Verification items for the finished model (mm, model axes). A direction names the side the tool comes from. Give positions to 0.01 mm unless a question says otherwise; leave off trailing zeros. Order: outer loops, then holes, each group sorted by start corner. A loop starts at its lowest first (then second) coordinate and runs counter-clockwise, first axis right, second up. Notation, with made-up numbers: (-7.5, 8.5) -> (6.5, 8.5) arc R20 ccw to (6.5, 32.5) -> close; hole circle Ø10 at (5, -18.75). An arc over 180 degrees is marked (long way). Write each question's results on one line, items separated by ' | '. Start each with the question number.
1. Set-up check for faces 1 (the face through (5.01, -13.43, 0.81)), 2 (the face through (7, -12.522, 1)): record each of +Z, -Z, +X, -X, +Y, -Y from which the full face is reachable in a straight line by a thin tool's end or side.
2. Depth check by flat-ended pin: pin 1 Ø1.7 at (x, y) = (-15.04, -11.37) entering from -Z; pin 2 Ø0.5 at (y, z) = (4, 1) entering from +X; pin 3 Ø1.3 at (x, y) = (0, -13.97) entering from -Z; pin 4 Ø0.5 at (x, z) = (8, 1) entering from +Y. Enter the tip coordinate at first touch or a pass-through.
3. Cross-section at D-D, the plane x = -9. Enter the section's corners in (y, z).
4. Cross-section at A-A, the plane x = 10.16. Enter the section's corners in (y, z), then the cut area to 3 significant figures.
5. Material ranges on L1, parallel to Y at x = 2.54, z = 1.2; L2, parallel to Y at x = -22.5, z = 1.3; L3, parallel to Y at x = -20.95, z = 0.85, recorded low to high. Write a range as from..to.
6. Cross-section at B-B, the plane y = -13.97. State how many separate pieces and enclosed holes the cut face has, then the cut area to 3 significant figures.
7. Mould release check, pull along X, two halves, no side actions. Record for faces 3 (the face through (-13.64, -11.31, 0.79)), 4 (the face through (-18, 16.51, 1)), 5 (the face through (25.4, -20, 1)): +X half, -X half, draft (parallel to the pull), parting line (faces both ways), or undercut.
Autodesk Inventor part; units mm, degrees
ref_plane "YZ Plane" through (0, 0, 0) normal (1, 0, 0) x (0, 1, 0)
ref_plane "XZ Plane" through (0, 0, 0) normal (0, 1, 0) x (-1, 0, 0)
ref_plane "XY Plane" through (0, 0, 0) normal (0, 0, 1) x (1, 0, 0)
sketch "Sketch1" plane through (0, 0, 0) normal (0, 0, 1) x (1, 0, 0)
  line L0 (-25.4, -16.51) -> (25.4, -16.51)
  line L1 (25.4, -16.51) -> (25.4, 16.51)
  line L2 (25.4, 16.51) -> (-25.4, 16.51)
  line L3 (-25.4, 16.51) -> (-25.4, -10.64)
  line L4 (-10.0076, 16.51) -> (-10.0076, -12.5222)
  line L5 (-10.0076, -12.5222) -> (25.4, -12.5222)
  line L6 (-25.4, -16.51) -> (-25.4, -26.4922)
  line L7 (-25.4, -26.4922) -> (25.4, -26.4922)
  line L8 (25.4, -26.4922) -> (25.4, -16.51)
  circle A0 centre (-2.54, -13.97) radius 0.5461
  circle A1 centre (2.54, -13.97) radius 0.5461
  circle A2 centre (7.62, -13.97) radius 0.5461
  circle A3 centre (-5.08, -7.62) radius 0.4445
  circle A4 centre (0, -7.62) radius 0.4445
  circle A5 centre (5.08, -7.62) radius 0.4445
  circle A6 centre (10.16, -7.62) radius 0.4445
  circle A7 centre (-5.08, 10.16) radius 0.4445
  circle A8 centre (0, 10.16) radius 0.4445
  circle A9 centre (5.08, 10.16) radius 0.4445
  circle A10 centre (10.16, 10.16) radius 0.4445
  circle A11 centre (12.7, 10.16) radius 0.4445
  circle A12 centre (7.62, 10.16) radius 0.4445
  circle A13 centre (2.54, 10.16) radius 0.4445
  circle A14 centre (-2.54, 10.16) radius 0.4445
  circle A15 centre (12.7, -7.62) radius 0.4445
  circle A16 centre (7.62, -7.62) radius 0.4445
  circle A17 centre (2.54, -7.62) radius 0.4445
  circle A18 centre (-2.54, -7.62) radius 0.4445
  circle A19 centre (10.16, -13.97) radius 0.5461
  circle A20 centre (5.08, -13.97) radius 0.5461
  circle A21 centre (0, -13.97) radius 0.5461
  circle A22 centre (-5.08, -13.97) radius 0.5461
  circle A23 centre (2.6924, -2.0574) radius 0.4445
  circle A24 centre (-2.3876, -2.0574) radius 0.4445
  circle A25 centre (-9.0424, 12.2174) radius 0.4445
  circle A26 centre (-14.1224, 12.2174) radius 0.4445
  circle A27 centre (-16.6624, 12.2174) radius 0.4445
  circle A28 centre (-11.5824, 12.2174) radius 0.4445
  circle A29 centre (-4.9276, -2.0574) radius 0.4445
  circle A30 centre (0.1524, -2.0574) radius 0.4445
  line L9 (-19.25, -14.29) -> (-25.4, -14.29)
  line L10 (-25.4, -14.29) -> (-25.4, -16.51)
  line L11 (-25.4, -10.64) -> (-19.25, -10.64)
  line L12 (-19.25, -10.64) -> (-19.25, -14.29)
  line L13 (-25.4, -14.29) -> (-25.4, -10.64)
  line L14 (-25.4, -10.64) -> (-19.25, -10.64)
  line L15 (-19.25, -10.64) -> (-19.25, -14.29)
  line L16 (-19.25, -14.29) -> (-25.4, -14.29)
  circle A31 centre (-23.81, 9.06) radius 0.4445
  circle A32 centre (17.14, 9.37) radius 0.4445
  circle A33 centre (19.68, 9.37) radius 0.4445
  circle A34 centre (-21.27, 9.06) radius 0.4445
  circle A35 centre (19.05, 13.97) radius 1.397
  point P0 (0, 0)
  dimension "d0" = 29.0322
  dimension "d1" = 35.4076
  dimension "d2" = 15.3924
  dimension "d3" = 13.97
extrude "Extrusion1" add sketch "Sketch1" along normal blind 1.6 contours L10 L9 L12 L11 L3 L2 L4 L5 L1 L0 | L0 L8 L7 L6 | L13 L11 L12 L9 | A0 | A1 | A2 | A19 | A20 | A21 | A22 | A26 | A27 | A28 | A31 | A34
sketch "Sketch2" plane through (0, 0, 1.6) normal (0, 0, 1) x (1, 0, 0)
  circle A0 centre (10.16, -13.97) radius 0.5461
  circle A1 centre (7.62, -13.97) radius 0.5461
  circle A2 centre (5.08, -13.97) radius 0.5461
  circle A3 centre (2.54, -13.97) radius 0.5461
  circle A4 centre (0, -13.97) radius 0.5461
  circle A5 centre (-2.54, -13.97) radius 0.5461
  circle A6 centre (-5.08, -13.97) radius 0.5461
  point P0 (0, 0)
extrude "Extrusion2" cut sketch "Sketch2" against normal blind 1.6
sketch "Sketch3" plane through (0, 0, 1.6) normal (0, 0, 1) x (1, 0, 0)
  line L0 (-25.4, 16.51) -> (-25.4, -26.4922) construction
  line L1 (-25.4, 12.11) -> (-10.0076, 12.11) construction
  line L2 (-10.0076, -12.5222) -> (-10.0076, 16.51) construction
  line L3 (-10.0076, 16.51) -> (-25.4, 16.51) construction
  line L4 (25.4, -12.5222) -> (-10.0076, -12.5222) construction
  line L5 (20.07, -12.5222) -> (20.07, -26.4922) construction
  line L6 (-25.4, -26.4922) -> (25.4, -26.4922) construction
  line L7 (25.4, -26.4922) -> (25.4, -12.5222) construction
  point P0 (0, 0)
  dimension "d8" = 4.4
  dimension "d9" = 5.33
sketch "Sketch4" plane through (0, 0, 1.6) normal (0, 0, 1) x (1, 0, 0)
  circle A0 centre (-23.49, -12.3622) radius 0.4445
  circle A1 centre (-20.95, -12.3622) radius 0.4445
  line L0 (-25.4, 16.51) -> (-25.4, -26.4922)
  line L1 (-25.4, -26.4922) -> (25.4, -26.4922)
  point P0 (0, 0)
  dimension "d10" = 0.889
  dimension "d11" = 0.889
  dimension "d12" = 1.91
  dimension "d13" = 2.54
  dimension "d14" = 0
  dimension "d15" = 14.13
extrude "Extrusion3" cut sketch "Sketch4" against normal blind 25.4
sketch "Sketch5" plane through (0, 0, 1.6) normal (0, 0, 1) x (1, 0, 0)
  circle A0 centre (-23.81, 9.06) radius 0.4445
  circle A1 centre (17.14, 9.37) radius 0.4445
  circle A2 centre (19.68, 9.37) radius 0.4445
  circle A3 centre (-21.27, 9.06) radius 0.4445
  line L0 (-25.4, -14.29) -> (-19.25, -14.29)
  line L1 (-19.25, -14.29) -> (-19.25, -10.64)
  line L2 (-19.25, -10.64) -> (-25.4, -10.64)
  line L3 (-25.4, 16.51) -> (-25.4, -10.64)
  line L4 (25.4, 16.51) -> (-25.4, 16.51)
  line L5 (25.4, -16.51) -> (25.4, 16.51)
  line L6 (-25.4, -16.51) -> (25.4, -16.51)
  line L7 (-25.4, -14.29) -> (-25.4, -16.51)
  circle A4 centre (-5.08, -13.97) radius 0.5461
  circle A5 centre (0, -13.97) radius 0.5461
  circle A6 centre (5.08, -13.97) radius 0.5461
  circle A7 centre (10.16, -13.97) radius 0.5461
  circle A8 centre (0.1524, -2.0574) radius 0.4445
  circle A9 centre (-4.9276, -2.0574) radius 0.4445
  circle A10 centre (-11.5824, 12.2174) radius 0.4445
  circle A11 centre (-16.6624, 12.2174) radius 0.4445
  circle A12 centre (-2.54, -7.62) radius 0.4445
  circle A13 centre (2.54, -7.62) radius 0.4445
  circle A14 centre (7.62, -7.62) radius 0.4445
  circle A15 centre (12.7, -7.62) radius 0.4445
  circle A16 centre (-2.54, 10.16) radius 0.4445
  circle A17 centre (2.54, 10.16) radius 0.4445
  circle A18 centre (7.62, 10.16) radius 0.4445
  circle A19 centre (12.7, 10.16) radius 0.4445
  circle A20 centre (10.16, 10.16) radius 0.4445
  circle A21 centre (5.08, 10.16) radius 0.4445
  circle A22 centre (0, 10.16) radius 0.4445
  circle A23 centre (-5.08, 10.16) radius 0.4445
  circle A24 centre (10.16, -7.62) radius 0.4445
  circle A25 centre (5.08, -7.62) radius 0.4445
  circle A26 centre (0, -7.62) radius 0.4445
  circle A27 centre (-5.08, -7.62) radius 0.4445
  circle A28 centre (-14.1224, 12.2174) radius 0.4445
  circle A29 centre (-9.0424, 12.2174) radius 0.4445
  circle A30 centre (-2.3876, -2.0574) radius 0.4445
  circle A31 centre (2.6924, -2.0574) radius 0.4445
  circle A32 centre (7.62, -13.97) radius 0.5461
  circle A33 centre (2.54, -13.97) radius 0.5461
  circle A34 centre (-2.54, -13.97) radius 0.5461
  circle A35 centre (19.05, 13.97) radius 1.397
  point P0 (0, 0)
extrude "Extrusion4" cut sketch "Sketch5" against normal blind 25.4 contours A0 | A3
sketch "Sketch6" plane through (0, 0, 1.6) normal (0, 0, 1) x (1, 0, 0)
  circle A0 centre (22.7674, -19.4372) radius 1.397
  point P0 (0, 0)
  dimension "d20" = 2.794
extrude "Extrusion5" cut sketch "Sketch6" against normal blind 25.4
sketch "Sketch7" plane through (0, 0, 0) normal (0, 0, -1) x (-1, 0, 0)
  circle A0 centre (15.0353, -11.3709) radius 1.397
  line L0 (24.1179, -7.9159) -> (10.0987, -7.9159)
  point P0 (0, 0)
  dimension "d23" = 2.794
  dimension "d24" = 3.455
extrude "Extrusion6" cut sketch "Sketch7" against normal blind 25.4
sketch "Sketch8" plane through (0, 0, 1.6) normal (0, 0, 1) x (1, 0, 0)
  circle A0 centre (-22.4387, 14.4799) radius 1.397
  point P0 (0, 0)
  dimension "d27" = 2.794
extrude "Extrusion7" cut sketch "Sketch8" against normal blind 25.4
properties part number "Control Board"
Results below:
1) face 1: +Z, -Z | face 2: +Z, -Z, +X, +Y
2) pin 1: passes through | pin 2: stops at x = -10.01 | pin 3: stops at z = 0 | pin 4: stops at y = -12.52
3) outline: (-26.49, 0) -> (-12.52, 0) -> (-12.52, 1.6) -> (-26.49, 1.6) -> close
4) outline: (-26.49, 0) -> (-14.52, 0) -> (-14.52, 1.6) -> (-26.49, 1.6) -> close; (-13.42, 0) -> (-12.52, 0) -> (-12.52, 1.6) -> (-13.42, 1.6) -> close | area: 20.6 mm²
5) L1: y = -26.49..-14.52, -13.42..-12.52 | L2: y = -26.49..13.08, 15.88..16.51 | L3: y = -26.49..-12.81, -11.92..8.75, 9.37..16.51
6) separate pieces: 8 | enclosed holes: 0 | area: 69.0 mm²
7) face 3: undercut | face 4: draft | face 5: +X half
